from build123d import *

# Parameters (mm, degrees)
F1_DEPTH = 1
F3_DEPTH = 25


with BuildPart() as f1:
    # F0 (on Front) → F1 (new body)
    with BuildSketch(Plane.XZ):
        Polygon((15.5, 19), (0, 0), (30.5, 0), (30.5, 19), align=None)
        Polygon((30.5, 19), (30.5, 0), (61, 0), (45.5, 19), align=None)
    extrude(amount=F1_DEPTH)

    # F2 (on face) → F3 (cut)
    with BuildSketch(Plane.XZ.offset(1)):
        with BuildLine():
            ThreePointArc((25.5, 16.75), (27.25, 15), (29, 16.75))
            ThreePointArc((29, 16.75), (27.25, 18.5), (25.5, 16.75))
        make_face()
        with BuildLine():
            ThreePointArc((35.5, 16.75), (33.75, 18.5), (32, 16.75))
            ThreePointArc((32, 16.75), (33.75, 15), (35.5, 16.75))
        make_face()
        with BuildLine():
            Line((35.5, 19), (32, 19))
            Line((32, 19), (32, 16.75))
            ThreePointArc((32, 16.75), (33.75, 18.5), (35.5, 16.75))
            Line((35.5, 16.75), (35.5, 19))
        make_face()
        with BuildLine():
            Line((29, 16.75), (29, 19))
            Line((29, 19), (25.5, 19))
            Line((25.5, 19), (25.5, 16.75))
            ThreePointArc((25.5, 16.75), (27.25, 18.5), (29, 16.75))
        make_face()
    extrude(amount=-F3_DEPTH, mode=Mode.SUBTRACT)


solid = f1.part
Work out the finished part from the listing and answer in its coordinate system (mm). A direction names the side the tool comes from. Give positions to 0.01 mm unless a question says otherwise; leave off trailing zeros. Loops run counter-clockwise (first coordinate to the right, second up) from the corner with the lowest first, then second, coordinate; pieces in that order, holes last. Notation, with made-up numbers: (-40, 66.5) - (-32, 66.5) arc R33 ccw to (-32, 98.5) - close; hole circle Ø1 at (13, 75.25). An arc over 180 degrees is marked (long way). Answer in a Markdown table with one row per item.
(1) For a pull along X with two mould halves and no side action, classify faces 3 (the face through (7.858, -0.493, 9.633)), 4 (the face through (29, -0.5, 17.9)), 5 (the face through (20.6, -0.5, 19)) as pulls with the +X half, pulls with the -X half, needs draft (parallel to the pull), parting line crosses it, or undercut.
Results list:
| item | result |
|---|---|
| face 3 | pulls with the -X half |
| face 4 | undercut |
| face 5 | needs draft |
(2) Section C-C (z = 9) is taken. Give the vertices of the cut face in (x, y), and give its area (3 significant figures).
Results list:
| item | result |
|---|---|
| outline | (7.34, -1) - (53.66, -1) - (53.66, 0) - (7.34, 0) - close |
| area | 46.3 mm² |
(3) Flat-ended cylindrical pins translate along their axes: pin 1 Ø0.5 at (y, z) = (-0.5, 17.5) entering from -X; pin 2 Ø0.5 at (y, z) = (-0.5, 18) entering from +X. Find the tip coordinate at first contact, or state that the pin passes through.
Results list:
| item | result |
|---|---|
| pin 1 | stops at x = 14.07 |
| pin 2 | stops at x = 46.52 |
(4) Section A-A (y = -0.3) is taken. Give the vertices of the cut face in (x, z), and give its area (3 significant figures).
Results list:
| item | result |
|---|---|
| outline | (0, 0) - (61, 0) - (45.5, 19) - (35.5, 19) - (35.5, 16.75) arc R1.75 cw to (32, 16.75) - (32, 19) - (29, 19) - (29, 16.75) arc R1.75 cw to (25.5, 16.75) - (25.5, 19) - (15.5, 19) - close |
| area | 839 mm² |
(5) Section B-B (x = 33.75) is taken. Give the vertices of the cut face in (y, z), and give its area (3 significant figures).
Results list:
| item | result |
|---|---|
| outline | (-1, 0) - (0, 0) - (0, 15) - (-1, 15) - close |
| area | 15.0 mm² |
(6) A tool of negligible diameter and unlimited length cuts with its end or side. For faces 1 (the face through (53.358, -0.493, 9.367)), 2 (the face through (35.5, -0.5, 17.9)), from which of +Z, -Z, +X, -X, +Y, -Y can it reach the whole face along a straight path? Write none if from no direction.
Results list:
| item | result |
|---|---|
| face 1 | +Z, +X, +Y, -Y |
| face 2 | +Z, +Y, -Y |
(7) Consider L1, parallel to X at y = -0.4, z = 17.5; L2, parallel to X at y = -0.4, z = 9.75; L3, parallel to Z at x = 33.5, y = -0.15. Determine where each line is inside the solid, lowest interval first. Write a range as [from, to].
Results list:
| item | result |
|---|---|
| L1 | x = [14.28, 25.5], [29, 32], [35.5, 46.72] |
| L2 | x = [7.95, 53.05] |
| L3 | z = [0, 15.02] |
